Part model, mm, in its own coordinate system. Face numbers are marked on the shaded views. Give positions to 0.01 mm unless a question says otherwise; leave off trailing zeros. Write each loop counter-clockwise with the first axis right and the second up, starting at its lowest first coordinate (ties: lowest second). Pieces come first, ordered by that corner, then holes. Notation, with made-up numbers: (73, 45) - (89, 45) arc R24 cw to (89, 74) - close; hole circle Ø2 at (-27.75, 26). An arc over 180 degrees is marked (long way). Answer in a Markdown table with one row per item. Add a question column.
1. Drop flat-ended pins along their axis: pin 1 Ø6 at (x, y) = (625.5, 95) entering from -Z; pin 2 Ø13.5 at (x, y) = (623, 100) entering from +Z; pin 3 Ø2 at (x, z) = (634.5, -16.5) entering from -Y. Give the stop position or say it passes through.
2. Band-saw the part on C-C on y = 98.5. Write the cut outline in (x, z).
3. Band-saw the part on D-D on x = 652. Write the cut outline in (y, z).
4. Probe line 1 along Z through (x, y) = (628.5, 110.25); line 2 along Z through (x, y) = (629.5, 94); line 3 along X through (y, z) = (105.75, -14). List the from-to ranges inside material, lowest first.
5. Band-saw the part on A-A on x = 618.5. Write the cut outline in (y, z), plus the area to 3 significant figures.
6. Pull direction X, two halves, no side cores. Call the marked faces 1, 2 and 3: released by +X, released by -X, zero draft, split by the parting line, or undercut.
7. Band-saw the part on B-B on z = -15. Write the cut outline in (x, y).
```python
from build123d import *

# Parameters (mm, degrees)
BOSS_EXTRUDE1_DEPTH = 21.59
SKETCH2_R           = 3.175
BOSS_EXTRUDE2_DEPTH = 2.54
BOSS_EXTRUDE3_START = 3.81
SKETCH3_R           = 3.175
BOSS_EXTRUDE3_DEPTH = 3.81
SKETCH6_R           = 3.175
BOSS_EXTRUDE4_DEPTH = 5.08


with BuildPart() as part:
    # Sketch1 → Boss-Extrude1 (new body)
    with BuildSketch(Plane.XY):
        with BuildLine():
            Line((629.598897849, 94.164329766), (616.850918015, 93.969698502))
            Line((616.850918015, 93.969698502), (616.909080854, 90.16014248))
            Line((616.909080854, 90.16014248), (640.914721516, 90.52665139))
            Line((640.914721516, 90.52665139), (640.60180544, 111.022062787))
            Line((640.60180544, 111.022062787), (634.252545404, 110.925124722))
            ThreePointArc((634.252545404, 110.925124722), (637.543945735, 103.811741783), (634.47123768, 96.601194079))
            ThreePointArc((634.47123768, 96.601194079), (632.210560309, 95.031876848), (629.598897849, 94.164329766))
        make_face()
    extrude(amount=-BOSS_EXTRUDE1_DEPTH)

    # Sketch2 → Boss-Extrude2 (add)
    with BuildSketch(Plane(origin=(0, 0, -19.05), x_dir=(-1, 0, 0), z_dir=(0, 0, -1))):
        with BuildLine():
            Line((-616.850918015, 93.969698502), (-616.596164778, 110.655553878))
            Line((-616.596164778, 110.655553878), (-634.252545404, 110.925124722))
            ThreePointArc((-634.252545404, 110.925124722), (-637.193249895, 101.082193986), (-629.598897849, 94.164329766))
            Line((-629.598897849, 94.164329766), (-616.850918015, 93.969698502))
        make_face()
        with Locations(Location((-627.893070479, 103.664395923, 0), (0, 0, 180))):
            Circle(SKETCH2_R, mode=Mode.SUBTRACT)
    extrude(amount=BOSS_EXTRUDE2_DEPTH)

    # Sketch3 → Boss-Extrude3 (add)
    # profile 1 of 2: a face of its own
    with BuildSketch(Plane.XY.offset(BOSS_EXTRUDE3_START)):
        with BuildLine():
            Line((634.252545404, 110.925124722), (616.596164778, 110.655553878))
            Line((616.596164778, 110.655553878), (616.850918015, 93.969698502))
            Line((616.850918015, 93.969698502), (629.598897849, 94.164329766))
            ThreePointArc((629.598897849, 94.164329766), (637.193249895, 101.082193986), (634.252545404, 110.925124722))
        make_face()
        with Locations((627.893070479, 103.664395923)):
            Circle(SKETCH3_R, mode=Mode.SUBTRACT)
    # profile 2 of 2: a face of its own
    with BuildSketch(Plane.XY.offset(BOSS_EXTRUDE3_START)):
        with BuildLine():
            Line((640.60180544, 111.022062787), (634.252545404, 110.925124722))
            ThreePointArc((634.252545404, 110.925124722), (637.193249895, 101.082193986), (629.598897849, 94.164329766))
            Line((629.598897849, 94.164329766), (616.850918015, 93.969698502))
            Line((616.850918015, 93.969698502), (616.909080854, 90.16014248))
            Line((616.909080854, 90.16014248), (640.914721516, 90.52665139))
            Line((640.914721516, 90.52665139), (640.60180544, 111.022062787))
        make_face()
    extrude(amount=-BOSS_EXTRUDE3_DEPTH)

    # Sketch6 → Boss-Extrude4 (add)
    with BuildSketch(Plane(origin=(1.009584834, 97.256608571, -1.08885119), x_dir=(0.9999461323694532, -0.01037876956131086, 0.00011619709707159731), z_dir=(0.010379419992088221, 0.9998834703189057, -0.011194347843893874))):
        Polygon((629.970445875, -30.830778579), (658.964231573, 31.318853688), (639.3986066, 40.446526963), (610.404820902, -21.703105303), align=None)
        with Locations(Location((623.94608709, -18.210508129, 0), (0, 0, 270))):
            Circle(SKETCH6_R, mode=Mode.SUBTRACT)
        with Locations(Location((645.422965385, 27.826256513, 0), (0, 0, 270))):
            Circle(SKETCH6_R, mode=Mode.SUBTRACT)
    extrude(amount=-BOSS_EXTRUDE4_DEPTH)


solid = part.part
```
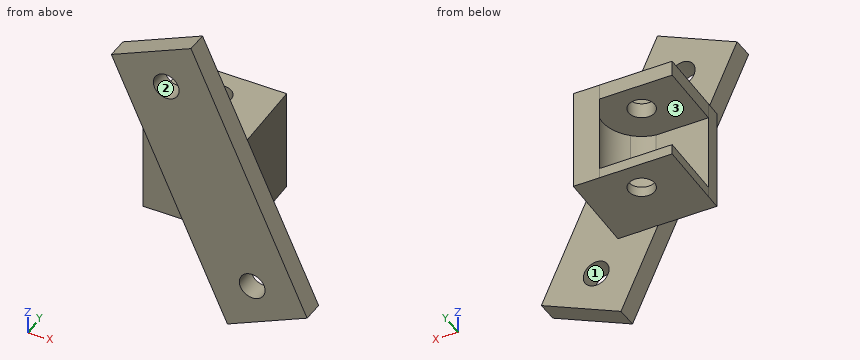
Values:
| question | item | result |
|---|---|---|
| 1 | pin 1 | stops at z = -21.59 |
| 1 | pin 2 | stops at z = 3.81 |
| 1 | pin 3 | stops at y = 85.41 |
| 2 | outline | (616.78, -21.59) - (640.79, -21.59) - (640.79, 3.81) - (616.78, 3.81) - (616.78, 0) - (636.05, 0) - (636.05, -19.05) - (616.78, -19.05) - close |
| 3 | outline | (85.03, -35.95) - (90.11, -36.03) - (90.34, -15.31) - (85.26, -15.37) - close |
| 4 | line 1 | z = -21.59 to -19.05, 0 to 3.81 |
| 4 | line 2 | z = -21.59 to 3.81 |
| 4 | line 3 | x = 637.32 to 640.68 |
| 5 | outline | (85.84, 5.37) - (90.92, 5.43) - (91.13, 24.01) - (86.05, 24.09) - close; (90.18, -21.59) - (110.68, -21.59) - (110.68, -19.05) - (93.99, -19.05) - (93.99, 0) - (110.68, 0) - (110.68, 3.81) - (90.18, 3.81) - close |
| 5 | area | 298 mm² |
| 6 | face 1 | undercut |
| 6 | face 2 | undercut |
| 6 | face 3 | zero draft |
| 7 | outline | (616.85, 93.97) - (616.91, 90.16) - (628.03, 90.33) - (628, 85.51) - (651.83, 85.26) - (651.85, 90.34) - (638.25, 90.49) - (640.91, 90.53) - (640.6, 111.02) - (634.25, 110.93) arc R9.65 cw to (629.6, 94.16) - close |
